Print and shaded views of the part. All mm, measured from the part's lowest x, y and z. Give positions to 0.01 mm unless a question says otherwise; leave off trailing zeros. Loops run counter-clockwise (first coordinate to the right, second up) from the corner with the lowest first, then second, coordinate; pieces in that order, holes last. Notation, with made-up numbers: M 52,25.25 L 87,25.25 A26 ccw 87,55.25 Z; hole C 59,-16 d5. An arc over 180 degrees is marked long. Put each result on its own line as item: value. Start each with the question number.
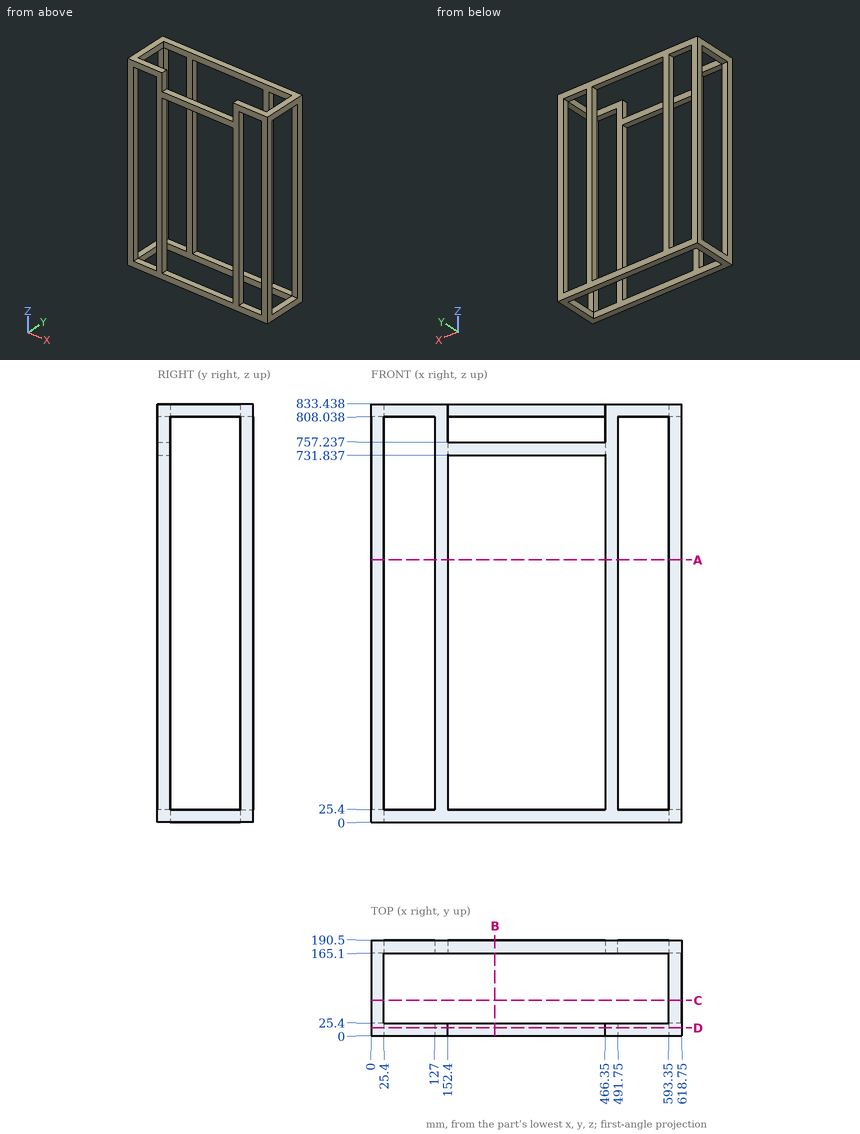
1) Band-saw the part on D-D on y = 16. Give the cut face in (x, z), then the cut area to 3 significant figures.
2) Pin check, flat tips, straight feed: pin 1 Ø7.5 at (x, y) = (536.5, 11.5) entering from -Z; pin 2 Ø4 at (x, z) = (494.5, 642.5) entering from -Y. Stop position of each tip, or through.
3) Band-saw the part on C-C on y = 71. Give the cut face in (x, z).
4) Band-saw the part on A-A on z = 523. State how many separate pieces and enclosed holes the cut face has, then the cut area to 3 significant figures.
5) Wall check: L1, parallel to X at y = 10, z = 539.5; L2, parallel to Y at x = 477.5, z = 378; L3, parallel to Z at x = 169, y = 21.5. Give the ranges that are in metal, low to high.
6) Band-saw the part on B-B on x = 246.5. Give the cut face in (y, z).
Evaluation:
1. outline: M 0,0 L 618.75,0 L 618.75,833.44 L 466.35,833.44 L 466.35,757.24 L 152.4,757.24 L 152.4,833.44 L 0,833.44 Z; hole M 25.4,25.4 L 127,25.4 L 127,808.04 L 25.4,808.04 Z; hole M 152.4,25.4 L 466.35,25.4 L 466.35,731.84 L 152.4,731.84 Z; hole M 491.75,25.4 L 593.35,25.4 L 593.35,808.04 L 491.75,808.04 Z
1. area: 111,000 mm2
2. pin 1: z = 0
2. pin 2: through
3. outline: M 0,0 L 25.4,0 L 25.4,25.4 L 0,25.4 Z; M 0,808.04 L 25.4,808.04 L 25.4,833.44 L 0,833.44 Z; M 593.35,0 L 618.75,0 L 618.75,25.4 L 593.35,25.4 Z; M 593.35,808.04 L 618.75,808.04 L 618.75,833.44 L 593.35,833.44 Z
4. separate pieces: 8
4. enclosed holes: 0
4. area: 5,160 mm2
5. L1: 0 to 25.4, 127 to 152.4, 466.35 to 491.75, 593.35 to 618.75
5. L2: 0 to 25.4, 165.1 to 190.5
5. L3: 0 to 25.4, 731.84 to 757.24
6. outline: M 0,0 L 25.4,0 L 25.4,25.4 L 0,25.4 Z; M 0,731.84 L 25.4,731.84 L 25.4,757.24 L 0,757.24 Z; M 165.1,0 L 190.5,0 L 190.5,25.4 L 165.1,25.4 Z; M 165.1,808.04 L 190.5,808.04 L 190.5,833.44 L 165.1,833.44 Z
